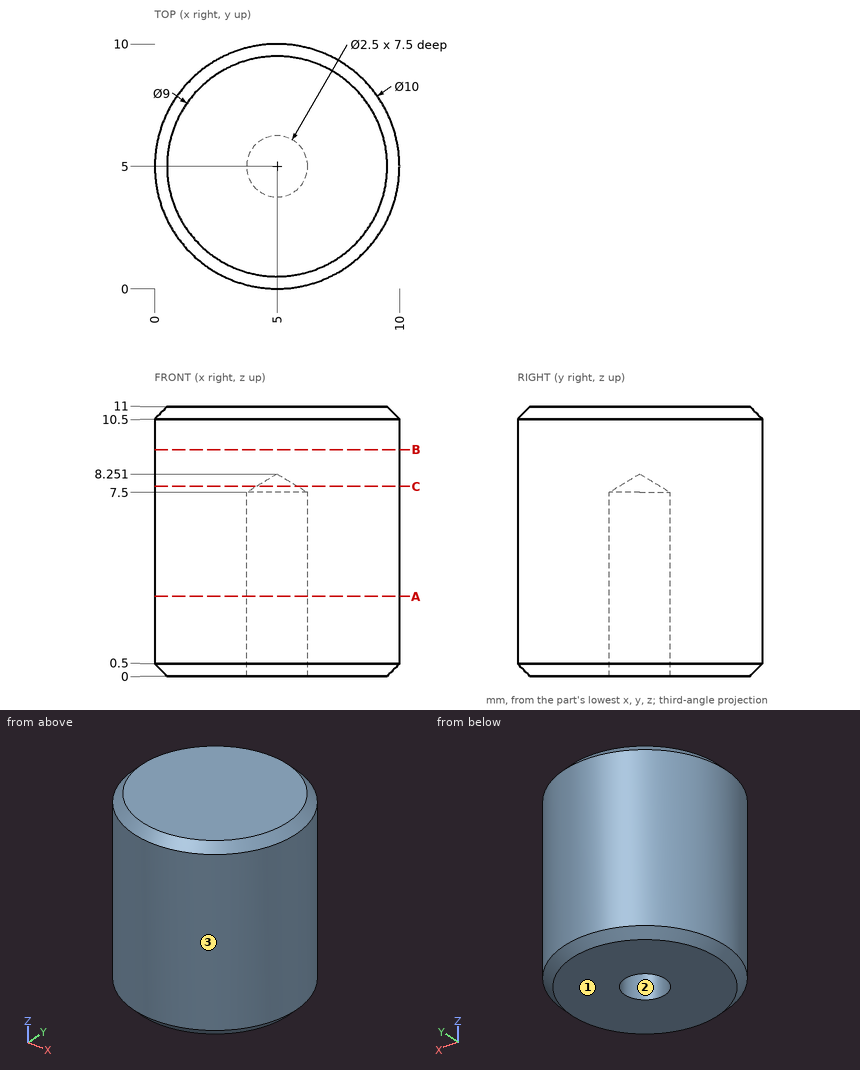
Can you work these out from the drawing? Everything is in mm from the part's minimum corner. Coordinates: 2 decimals unless noted, no trailing zeros. Write each loop counter-clockwise with the first axis right and the second up, starting at its lowest first coordinate (ties: lowest second). Pieces come first, ordered by that corner, then holes. Notation, with made-up numbers: (80.25, 82.5) -> (115.25, 82.5) arc R25 cw to (115.25, 100.5) -> close; hole circle Ø5 at (59, -32). An arc over 180 degrees is marked (long way). Write item = value, one per line.
(1) Imagine slicing it at C-C (z = 7.75). Please give me the cut outline in (x, y).
Verdict:
outline = circle Ø10 at (5, 5); hole circle Ø1.67 at (5, 5)
(2) Imagine slicing it at B-B (z = 9.25). Please give me the cut outline in (x, y), and give its area (3 significant figures).
Verdict:
outline = circle Ø10 at (5, 5)
area = 78.5 mm^2
(3) Thinking about a two-plate mould opening in Y: for the marked faces 1, 2 and 3, which applies, +Y half, -Y half, draft (parallel to the pull), parting line (faces both ways), or undercut?
Verdict:
face_1 = draft
face_2 = undercut
face_3 = parting line
(4) For pin 1 (4 mm diameter, centred on y = 2.5, z = 10, fed in from -X) (3 decimals); pin 2 (1 mm diameter, centred on y = 8, z = 9.5, fed in from -X); pin 3 (4 mm diameter, centred on y = 2.5, z = 9.5, fed in from +X) (3 decimals), each with a flat end and sliding along its axis, tell me the tip position at first contact or that it passes through.
Verdict:
pin_1 = 0.025
pin_2 = 0.67
pin_3 = 9.975
(5) Imagine slicing it at A-A (z = 3.25). Please give me the cut outline in (x, y), and give its area (3 significant figures).
Verdict:
outline = circle Ø10 at (5, 5); hole circle Ø2.5 at (5, 5)
area = 73.6 mm^2
(6) If I drill on probe 1 along Y at (x, z) = (5, 4.25); probe 2 along X at (y, z) = (5.25, 7); probe 3 along Y at (x, z) = (4, 1.5), over which ranges is the centre line in solid material (lowest first)?
Verdict:
probe_1 = 0 to 3.75, 6.25 to 10
probe_2 = 0.01 to 3.78, 6.22 to 9.99
probe_3 = 0.1 to 4.25, 5.75 to 9.9
